from build123d import *

# Parameters (mm, degrees)
SKETCH3_W           = 158.75
SKETCH3_H           = 109.9058
BOSS_EXTRUDE4_DEPTH = 19.05
CUT_EXTRUDE7_DEPTH  = 12.7
CUT_EXTRUDE8_DEPTH  = 7.35
CUT_EXTRUDE9_DEPTH  = 5.08


with BuildPart() as part:
    # Sketch3 → Boss-Extrude4 (new body)
    with BuildSketch(Plane(origin=(0, 0, 0), x_dir=(1, 0, 0), z_dir=(0, 1, 0))):
        with Locations((79.375, 54.9529)):
            Rectangle(SKETCH3_W, SKETCH3_H)
    extrude(amount=-BOSS_EXTRUDE4_DEPTH)

    # Sketch3<12> → Cut-Extrude7 (cut)
    with BuildSketch(Plane(origin=(0, 0, 0), x_dir=(1, 0, 0), z_dir=(0, 1, 0))):
        with BuildLine():
            ThreePointArc((82.55, 21.59), (83.293948776, 19.793948776), (85.09, 19.05))
            Line((85.09, 19.05), (88.4842, 19.05))
            Line((88.4842, 19.05), (88.4842, 8.89))
            ThreePointArc((88.4842, 8.89), (89.228148776, 7.093948776), (91.0242, 6.35))
            Line((91.0242, 6.35), (94.885, 6.35))
            ThreePointArc((94.885, 6.35), (96.681051224, 7.093948776), (97.425, 8.89))
            Line((97.425, 8.89), (97.425, 19.05))
            Line((97.425, 19.05), (99.425, 19.05))
            Line((99.425, 19.05), (99.425, 8.89))
            ThreePointArc((99.425, 8.89), (100.168948776, 7.093948776), (101.965, 6.35))
            Line((101.965, 6.35), (105.8258, 6.35))
            ThreePointArc((105.8258, 6.35), (107.621851224, 7.093948776), (108.3658, 8.89))
            Line((108.3658, 8.89), (108.3658, 19.05))
            Line((108.3658, 19.05), (111.76, 19.05))
            ThreePointArc((111.76, 19.05), (113.556051224, 19.793948776), (114.3, 21.59))
            Line((114.3, 21.59), (114.3, 101.0158))
            ThreePointArc((114.3, 101.0158), (113.556051224, 102.811851224), (111.76, 103.5558))
            Line((111.76, 103.5558), (85.09, 103.5558))
            ThreePointArc((85.09, 103.5558), (83.293948776, 102.811851224), (82.55, 101.0158))
            Line((82.55, 101.0158), (82.55, 21.59))
        make_face()
        with BuildLine():
            Line((6.35, 101.0158), (6.35, 21.59))
            ThreePointArc((6.35, 21.59), (7.093948776, 19.793948776), (8.89, 19.05))
            Line((8.89, 19.05), (12.2842, 19.05))
            Line((12.2842, 19.05), (12.2842, 8.89))
            ThreePointArc((12.2842, 8.89), (13.028148776, 7.093948776), (14.8242, 6.35))
            Line((14.8242, 6.35), (18.685, 6.35))
            ThreePointArc((18.685, 6.35), (20.481051224, 7.093948776), (21.225, 8.89))
            Line((21.225, 8.89), (21.225, 19.05))
            Line((21.225, 19.05), (23.225, 19.05))
            Line((23.225, 19.05), (23.225, 8.89))
            ThreePointArc((23.225, 8.89), (23.968948776, 7.093948776), (25.765, 6.35))
            Line((25.765, 6.35), (29.6258, 6.35))
            ThreePointArc((29.6258, 6.35), (31.421851224, 7.093948776), (32.1658, 8.89))
            Line((32.1658, 8.89), (32.1658, 19.05))
            Line((32.1658, 19.05), (35.56, 19.05))
            ThreePointArc((35.56, 19.05), (37.356051224, 19.793948776), (38.1, 21.59))
            Line((38.1, 21.59), (38.1, 101.0158))
            ThreePointArc((38.1, 101.0158), (37.356051224, 102.811851224), (35.56, 103.5558))
            Line((35.56, 103.5558), (8.89, 103.5558))
            ThreePointArc((8.89, 103.5558), (7.093948776, 102.811851224), (6.35, 101.0158))
        make_face()
        with BuildLine():
            ThreePointArc((46.99, 103.5558), (45.193948776, 102.811851224), (44.45, 101.0158))
            Line((44.45, 101.0158), (44.45, 21.59))
            ThreePointArc((44.45, 21.59), (45.193948776, 19.793948776), (46.99, 19.05))
            Line((46.99, 19.05), (50.3842, 19.05))
            Line((50.3842, 19.05), (50.3842, 8.89))
            ThreePointArc((50.3842, 8.89), (51.128148776, 7.093948776), (52.9242, 6.35))
            Line((52.9242, 6.35), (56.785, 6.35))
            ThreePointArc((56.785, 6.35), (58.581051224, 7.093948776), (59.325, 8.89))
            Line((59.325, 8.89), (59.325, 19.05))
            Line((59.325, 19.05), (61.325, 19.05))
            Line((61.325, 19.05), (61.325, 8.89))
            ThreePointArc((61.325, 8.89), (62.068948776, 7.093948776), (63.865, 6.35))
            Line((63.865, 6.35), (67.7258, 6.35))
            ThreePointArc((67.7258, 6.35), (69.521851224, 7.093948776), (70.2658, 8.89))
            Line((70.2658, 8.89), (70.2658, 19.05))
            Line((70.2658, 19.05), (73.66, 19.05))
            ThreePointArc((73.66, 19.05), (75.456051224, 19.793948776), (76.2, 21.59))
            Line((76.2, 21.59), (76.2, 101.0158))
            ThreePointArc((76.2, 101.0158), (75.456051224, 102.811851224), (73.66, 103.5558))
            Line((73.66, 103.5558), (46.99, 103.5558))
        make_face()
        with BuildLine():
            ThreePointArc((120.65, 21.59), (121.393948776, 19.793948776), (123.19, 19.05))
            Line((123.19, 19.05), (126.5842, 19.05))
            Line((126.5842, 19.05), (126.5842, 8.89))
            ThreePointArc((126.5842, 8.89), (127.328148776, 7.093948776), (129.1242, 6.35))
            Line((129.1242, 6.35), (132.985, 6.35))
            ThreePointArc((132.985, 6.35), (134.781051224, 7.093948776), (135.525, 8.89))
            Line((135.525, 8.89), (135.525, 19.05))
            Line((135.525, 19.05), (137.525, 19.05))
            Line((137.525, 19.05), (137.525, 8.89))
            ThreePointArc((137.525, 8.89), (138.268948776, 7.093948776), (140.065, 6.35))
            Line((140.065, 6.35), (143.9258, 6.35))
            ThreePointArc((143.9258, 6.35), (145.721851224, 7.093948776), (146.4658, 8.89))
            Line((146.4658, 8.89), (146.4658, 19.05))
            Line((146.4658, 19.05), (149.86, 19.05))
            ThreePointArc((149.86, 19.05), (151.656051224, 19.793948776), (152.4, 21.59))
            Line((152.4, 21.59), (152.4, 101.0158))
            ThreePointArc((152.4, 101.0158), (151.656051224, 102.811851224), (149.86, 103.5558))
            Line((149.86, 103.5558), (123.19, 103.5558))
            ThreePointArc((123.19, 103.5558), (121.393948776, 102.811851224), (120.65, 101.0158))
            Line((120.65, 101.0158), (120.65, 21.59))
        make_face()
    extrude(amount=-CUT_EXTRUDE7_DEPTH, mode=Mode.SUBTRACT)

    # Sketch5 → Cut-Extrude8 (cut, through all)
    with BuildSketch(Plane(origin=(0, -12.7, 0), x_dir=(1, 0, 0), z_dir=(0, 1, 0))):
        with BuildLine():
            Line((25.4, 87.6808), (25.4, 81.3308))
            ThreePointArc((25.4, 81.3308), (22.225, 78.1558), (19.05, 81.3308))
            Line((19.05, 81.3308), (19.05, 87.6808))
            ThreePointArc((19.05, 87.6808), (22.225, 90.8558), (25.4, 87.6808))
        make_face()
        with BuildLine():
            Line((25.4, 41.275), (25.4, 34.925))
            ThreePointArc((25.4, 34.925), (22.225, 31.75), (19.05, 34.925))
            Line((19.05, 34.925), (19.05, 41.275))
            ThreePointArc((19.05, 41.275), (22.225, 44.45), (25.4, 41.275))
        make_face()
        with BuildLine():
            Line((57.15, 34.925), (57.15, 41.275))
            ThreePointArc((57.15, 41.275), (60.325, 44.45), (63.5, 41.275))
            Line((63.5, 41.275), (63.5, 34.925))
            ThreePointArc((63.5, 34.925), (60.325, 31.75), (57.15, 34.925))
        make_face()
        with BuildLine():
            Line((57.15, 81.3308), (57.15, 87.6808))
            ThreePointArc((57.15, 87.6808), (60.325, 90.8558), (63.5, 87.6808))
            Line((63.5, 87.6808), (63.5, 81.3308))
            ThreePointArc((63.5, 81.3308), (60.325, 78.1558), (57.15, 81.3308))
        make_face()
        with BuildLine():
            Line((101.6, 87.6808), (101.6, 81.3308))
            ThreePointArc((101.6, 81.3308), (98.425, 78.1558), (95.25, 81.3308))
            Line((95.25, 81.3308), (95.25, 87.6808))
            ThreePointArc((95.25, 87.6808), (98.425, 90.8558), (101.6, 87.6808))
        make_face()
        with BuildLine():
            Line((101.6, 41.275), (101.6, 34.925))
            ThreePointArc((101.6, 34.925), (98.425, 31.75), (95.25, 34.925))
            Line((95.25, 34.925), (95.25, 41.275))
            ThreePointArc((95.25, 41.275), (98.425, 44.45), (101.6, 41.275))
        make_face()
        with BuildLine():
            Line((139.7, 41.275), (139.7, 34.925))
            ThreePointArc((139.7, 34.925), (136.525, 31.75), (133.35, 34.925))
            Line((133.35, 34.925), (133.35, 41.275))
            ThreePointArc((133.35, 41.275), (136.525, 44.45), (139.7, 41.275))
        make_face()
        with BuildLine():
            Line((139.7, 87.6808), (139.7, 81.3308))
            ThreePointArc((139.7, 81.3308), (136.525, 78.1558), (133.35, 81.3308))
            Line((133.35, 81.3308), (133.35, 87.6808))
            ThreePointArc((133.35, 87.6808), (136.525, 90.8558), (139.7, 87.6808))
        make_face()
    extrude(amount=-CUT_EXTRUDE8_DEPTH, mode=Mode.SUBTRACT)

    # Sketch7 → Cut-Extrude9 (cut)
    with BuildSketch(Plane(origin=(0, 0, 0), x_dir=(1, 0, 0), z_dir=(0, 1, 0))):
        with BuildLine():
            Line((2.8575, 45.72), (3.4925, 45.72))
            ThreePointArc((3.4925, 45.72), (4.390525612, 45.348025612), (4.7625, 44.45))
            Line((4.7625, 44.45), (4.7625, 39.37))
            ThreePointArc((4.7625, 39.37), (4.390525612, 38.471974388), (3.4925, 38.1))
            Line((3.4925, 38.1), (2.8575, 38.1))
            ThreePointArc((2.8575, 38.1), (1.959474388, 38.471974388), (1.5875, 39.37))
            Line((1.5875, 39.37), (1.5875, 44.45))
            ThreePointArc((1.5875, 44.45), (1.959474388, 45.348025612), (2.8575, 45.72))
        make_face()
        with BuildLine():
            Line((153.9875, 44.45), (153.9875, 39.37))
            ThreePointArc((153.9875, 39.37), (154.359474388, 38.471974388), (155.2575, 38.1))
            Line((155.2575, 38.1), (155.8925, 38.1))
            ThreePointArc((155.8925, 38.1), (156.790525612, 38.471974388), (157.1625, 39.37))
            Line((157.1625, 39.37), (157.1625, 44.45))
            ThreePointArc((157.1625, 44.45), (156.790525612, 45.348025612), (155.8925, 45.72))
            Line((155.8925, 45.72), (155.2575, 45.72))
            ThreePointArc((155.2575, 45.72), (154.359474388, 45.348025612), (153.9875, 44.45))
        make_face()
    extrude(amount=-CUT_EXTRUDE9_DEPTH, mode=Mode.SUBTRACT)


solid = part.part
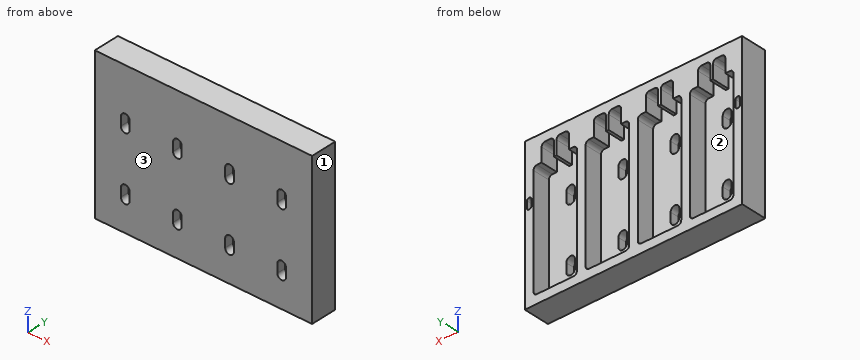
Design review of the part built by this model. Coordinates are the model's own, in mm. Face numbers are marked on the shaded views. Round coordinates to 2 decimals unless told otherwise and drop trailing zeros. Write each loop counter-clockwise with the first axis right and the second up, starting at its lowest first coordinate (ties: lowest second). Pieces come first, ordered by that corner, then holes. Notation, with made-up numbers: M 35.5,8.5 L 88.5,8.5 A25 cw 88.5,23.5 Z; hole C 30.25,57.5 d3. An arc over 180 degrees is marked long. One line per item, written item: value. Start each with the question number.
1. Take a section at A-A on x = 93. State the section outline as (y, z) points, then the cut area to 3 significant figures.
2. Take a section at B-B on z = -63. State the section outline as (x, y) points, then the cut area to 3 significant figures.
3. To check wall thickness, follow probe 1 along X at (y, z) = (-9, -48.5); probe 2 along X at (y, z) = (-17.5, -83); probe 3 along Z at (x, y) = (53.5, -5). State the ranges of each line that lie inside material, in increasing order. Write a range as from..to.
4. Draft analysis for pull direction X (two halves, no side actions). For the marked faces 1, 2 and 3, state which applies: pulls with the +X half, pulls with the -X half, needs draft (parallel to the pull), parting line crosses it, or undercut.
5. Take a section at C-C on y = -15.25. State how many separate pieces and enclosed holes the cut face has, then the cut area to 3 significant figures.
Computed:
1. outline: M -19.05,-109.91 L 0,-109.91 L 0,-103.56 L -12.7,-103.56 L -12.7,-6.35 L 0,-6.35 L 0,0 L -19.05,0 Z
1. area: 859 mm²
2. outline: M 0,-19.05 L 158.75,-19.05 L 158.75,0 L 152.4,0 L 152.4,-12.7 L 120.65,-12.7 L 120.65,0 L 114.3,0 L 114.3,-12.7 L 82.55,-12.7 L 82.55,0 L 76.2,0 L 76.2,-12.7 L 44.45,-12.7 L 44.45,0 L 38.1,0 L 38.1,-12.7 L 6.35,-12.7 L 6.35,0 L 0,0 Z
2. area: 1,410 mm²
3. probe 1: x = 0..6.35, 38.1..44.45, 76.2..82.55, 114.3..120.65, 152.4..158.75
3. probe 2: x = 0..19.05, 25.4..57.15, 63.5..95.25, 101.6..133.35, 139.7..158.75
3. probe 3: z = -109.91..-103.56, -6.35..0
4. face 1: pulls with the +X half
4. face 2: undercut
4. face 3: needs draft
5. separate pieces: 1
5. enclosed holes: 8
5. area: 16,900 mm²
